Can you work these out from the model? Positions are in its coordinate system, mm. Coordinates: 2 decimals unless noted, no trailing zeros. Return JSON: item names as keys, results as strings. Group by question number.
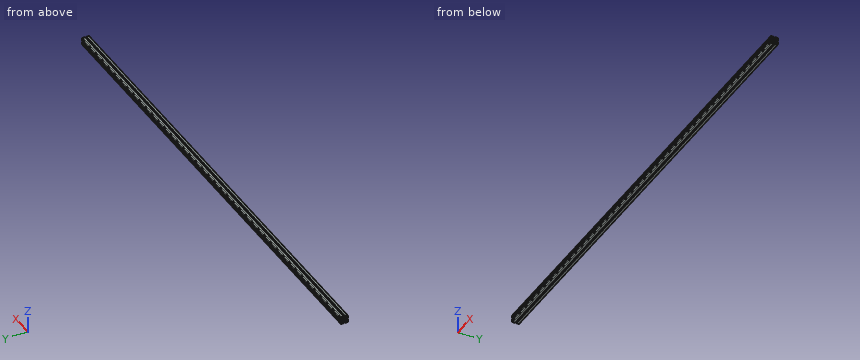
```python
from build123d import *

# Parameters (mm, degrees)
SKETCH_3_R          = 3.4
EXTRUDE_1_DEPTH     = 2622
CUT_EXTRUDE_3_DEPTH = 3297


with BuildPart() as part:
    # 草图3 → 凸台-拉伸1 (new body)
    with BuildSketch(Plane(origin=(0, 0, 0), x_dir=(0, 0, -1), z_dir=(1, 0, 0))):
        with BuildLine():
            Line((-15.5, -20), (-4.5, -20))
            Line((-4.5, -20), (-4.5, -19.5))
            Line((-4.5, -19.5), (-4.1, -19.5))
            Line((-4.1, -19.5), (-4.1, -16.2))
            Line((-4.1, -16.2), (-6.4, -16.2))
            Line((-6.4, -16.2), (-6.4, -18.2))
            Line((-6.4, -18.2), (-10.25, -18.2))
            Line((-10.25, -18.2), (-10.25, -11.522792206))
            Line((-10.25, -11.522792206), (-5.479130441, -6.751922647))
            Line((-5.479130441, -6.751922647), (5.479130441, -6.751922647))
            Line((5.479130441, -6.751922647), (10.25, -11.522792206))
            Line((10.25, -11.522792206), (10.25, -18.2))
            Line((10.25, -18.2), (6.4, -18.2))
            Line((6.4, -18.2), (6.4, -16.2))
            Line((6.4, -16.2), (4.1, -16.2))
            Line((4.1, -16.2), (4.1, -19.5))
            Line((4.1, -19.5), (4.5, -19.5))
            Line((4.5, -19.5), (4.5, -20))
            Line((4.5, -20), (15.5, -20))
            ThreePointArc((15.5, -20), (18.681980515, -18.681980515), (20, -15.5))
            Line((20, -15.5), (20, -4.5))
            Line((20, -4.5), (19.5, -4.5))
            Line((19.5, -4.5), (19.5, -4.1))
            Line((19.5, -4.1), (16.2, -4.1))
            Line((16.2, -4.1), (16.2, -6.4))
            Line((16.2, -6.4), (18.2, -6.4))
            Line((18.2, -6.4), (18.2, -10.25))
            Line((18.2, -10.25), (11.522792206, -10.25))
            Line((11.522792206, -10.25), (6.751922647, -5.479130441))
            Line((6.751922647, -5.479130441), (6.751922647, 5.479130441))
            Line((6.751922647, 5.479130441), (11.522792206, 10.25))
            Line((11.522792206, 10.25), (18.2, 10.25))
            Line((18.2, 10.25), (18.2, 6.4))
            Line((18.2, 6.4), (16.2, 6.4))
            Line((16.2, 6.4), (16.2, 4.1))
            Line((16.2, 4.1), (19.5, 4.1))
            Line((19.5, 4.1), (19.5, 4.5))
            Line((19.5, 4.5), (20, 4.5))
            Line((20, 4.5), (20, 15.5))
            ThreePointArc((20, 15.5), (18.681980515, 18.681980515), (15.5, 20))
            Line((15.5, 20), (4.5, 20))
            Line((4.5, 20), (4.5, 19.5))
            Line((4.5, 19.5), (4.1, 19.5))
            Line((4.1, 19.5), (4.1, 16.2))
            Line((4.1, 16.2), (6.4, 16.2))
            Line((6.4, 16.2), (6.4, 18.2))
            Line((6.4, 18.2), (10.25, 18.2))
            Line((10.25, 18.2), (10.25, 11.522792206))
            Line((10.25, 11.522792206), (5.479130441, 6.751922647))
            Line((5.479130441, 6.751922647), (-5.479130441, 6.751922647))
            Line((-5.479130441, 6.751922647), (-10.25, 11.522792206))
            Line((-10.25, 11.522792206), (-10.25, 18.2))
            Line((-10.25, 18.2), (-6.4, 18.2))
            Line((-6.4, 18.2), (-6.4, 16.2))
            Line((-6.4, 16.2), (-4.1, 16.2))
            Line((-4.1, 16.2), (-4.1, 19.5))
            Line((-4.1, 19.5), (-4.5, 19.5))
            Line((-4.5, 19.5), (-4.5, 20))
            Line((-4.5, 20), (-15.5, 20))
            ThreePointArc((-15.5, 20), (-18.681980515, 18.681980515), (-20, 15.5))
            Line((-20, 15.5), (-20, 4.5))
            Line((-20, 4.5), (-19.5, 4.5))
            Line((-19.5, 4.5), (-19.5, 4.1))
            Line((-19.5, 4.1), (-16.2, 4.1))
            Line((-16.2, 4.1), (-16.2, 6.4))
            Line((-16.2, 6.4), (-18.2, 6.4))
            Line((-18.2, 6.4), (-18.2, 10.25))
            Line((-18.2, 10.25), (-11.522792206, 10.25))
            Line((-11.522792206, 10.25), (-6.751922647, 5.479130441))
            Line((-6.751922647, 5.479130441), (-6.751922647, -5.479130441))
            Line((-6.751922647, -5.479130441), (-11.522792206, -10.25))
            Line((-11.522792206, -10.25), (-18.2, -10.25))
            Line((-18.2, -10.25), (-18.2, -6.4))
            Line((-18.2, -6.4), (-16.2, -6.4))
            Line((-16.2, -6.4), (-16.2, -4.1))
            Line((-16.2, -4.1), (-19.5, -4.1))
            Line((-19.5, -4.1), (-19.5, -4.5))
            Line((-19.5, -4.5), (-20, -4.5))
            Line((-20, -4.5), (-20, -15.5))
            ThreePointArc((-20, -15.5), (-18.681980515, -18.681980515), (-15.5, -20))
        make_face()
        Circle(SKETCH_3_R, mode=Mode.SUBTRACT)
    extrude(amount=EXTRUDE_1_DEPTH)

    # 草图4 → 切除-拉伸3 (cut)
    with BuildSketch(Plane(origin=(2622, -20, 15.5), x_dir=(0, 0, 1), z_dir=(-1, 0, 0))):
        with BuildLine():
            Line((-3.75, 31.75), (3, 31.75))
            Line((3, 31.75), (3, 35.5))
            ThreePointArc((3, 35.5), (2.121320344, 37.621320344), (0, 38.5))
            Line((0, 38.5), (-3.75, 38.5))
            Line((-3.75, 38.5), (-3.75, 31.75))
        make_face()
        with BuildLine():
            Line((-3.75, 8.25), (-3.75, 1.5))
            Line((-3.75, 1.5), (0, 1.5))
            ThreePointArc((0, 1.5), (2.121320344, 2.378679656), (3, 4.5))
            Line((3, 4.5), (3, 8.25))
            Line((3, 8.25), (-3.75, 8.25))
        make_face()
        with BuildLine():
            Line((-27.25, 8.25), (-34, 8.25))
            Line((-34, 8.25), (-34, 4.5))
            ThreePointArc((-34, 4.5), (-33.121320344, 2.378679656), (-31, 1.5))
            Line((-31, 1.5), (-27.25, 1.5))
            Line((-27.25, 1.5), (-27.25, 8.25))
        make_face()
        with BuildLine():
            Line((-27.25, 31.75), (-27.25, 38.5))
            Line((-27.25, 38.5), (-31, 38.5))
            ThreePointArc((-31, 38.5), (-33.121320344, 37.621320344), (-34, 35.5))
            Line((-34, 35.5), (-34, 31.75))
            Line((-34, 31.75), (-27.25, 31.75))
        make_face()
    extrude(amount=CUT_EXTRUDE_3_DEPTH, mode=Mode.SUBTRACT)


solid = part.part
```
1) Suppose I cut it at A-A, the plane x = 1307. Give the number of separate pieces and of enclosed holes in the cut face, then the cut area to 3 significant figures.
2) If I drill on line 1 (Z direction, x = 2481.5, y = 13); line 2 (Y direction, x = 1402, z = -18), over which ranges is the centre line in solid material (lowest first)? Write a range as from..to.
3) For pin 1 (2.5 mm diameter, centred on x = 1693.5, z = 17.5, fed in from -Y); pin 2 (12 mm diameter, centred on x = 1957, z = -2.5, fed in from -Y); pin 3 (3.5 mm diameter, centred on x = 1245.5, z = -1.5, fed in from -Y); pin 4 (3.5 mm diameter, centred on x = 1806, y = -17.5, fed in from -Z), each with a flat end and sliding along its axis, tell me the tip position at first contact or that it passes through.
Returned:
{
 "1": {"separate pieces": "1", "enclosed holes": "5", "area": "500 mm²"},
 "2": {"line 1": "z = -20..-18.5, -11.75..-10.25, 10.25..11.75, 18.5..20", "line 2": "y = -19.24..-17.16, -11.75..-10.25, -6.4..-4.1, 4.1..6.4, 10.25..11.75, 17.16..19.24"},
 "3": {"pin 1": "stops at y = -19.94", "pin 2": "stops at y = -20", "pin 3": "stops at y = -6.75", "pin 4": "stops at z = -19.99"}
}
